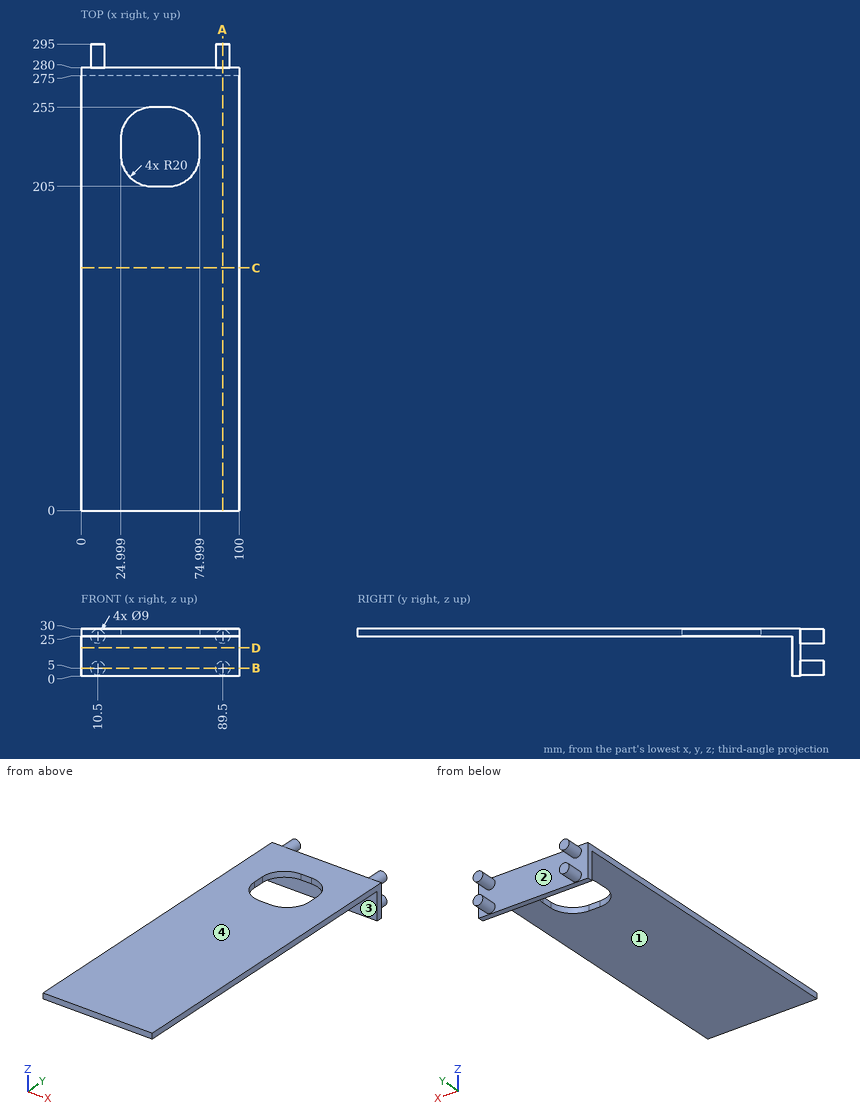
Study the drawing (mm; zero at the part's minimum x, y, z) and answer. A direction names the side the tool comes from. Round coordinates to 2 decimals unless told otherwise and drop trailing zeros. Write each loop counter-clockwise with the first axis right and the second up, starting at its lowest first coordinate (ties: lowest second). Pieces come first, ordered by that corner, then holes. Notation, with made-up numbers: (8, 16.5) -> (37, 16.5) arc R26 cw to (37, 55.5) -> close; hole circle Ø6 at (24.5, -28.5). An arc over 180 degrees is marked (long way). Write item = value, one per line.
1) Straight lines are drawn through the part: line 1 along Y through (x, z) = (51, 26.5); line 2 along X through (y, z) = (227.5, 28.75); line 3 along Z through (x, y) = (91.5, 106). For each, find the intervals that lie inside material, in ascending order. Write a range as [from, to].
Check values:
line_1 = [0, 205], [255, 280]
line_2 = [0, 25], [75, 100]
line_3 = [25, 30]
2) Section C-C on y = 153.5 is taken. Write down the section's boundary in (x, z).
Check values:
outline = (0, 25) -> (100, 25) -> (100, 30) -> (0, 30) -> close
3) Section B-B on z = 5 is taken. Write down the section's boundary in (x, y), plus the area to 3 significant figures.
Check values:
outline = (0, 275) -> (100, 275) -> (100, 280) -> (94, 280) -> (94, 295) -> (85, 295) -> (85, 280) -> (15, 280) -> (15, 295) -> (6, 295) -> (6, 280) -> (0, 280) -> close
area = 770 mm²
4) Given pin 1 (2 mm diameter, centred on x = 53.5, y = 34, fed in from -Z); pin 2 (8 mm diameter, centred on x = 33.5, z = 15, fed in from +Y); pin 3 (10 mm diameter, centred on x = 37.5, z = 5.5, fed in from -Y), each flat-ended and moving along its own axis, determine where each tip first touches the part or whether it passes through.
Check values:
pin_1 = 25
pin_2 = 280
pin_3 = 275
5) For a pull along X with two mould halves and no side action, classify the marked faces 1 and 2 as released by +X, released by -X, zero draft, split by the parting line, or undercut.
Check values:
face_1 = zero draft
face_2 = undercut
6) Section D-D on z = 17.75 is taken. Write down the section's boundary in (x, y), plus the area to 3 significant figures.
Check values:
outline = (0, 275) -> (100, 275) -> (100, 280) -> (0, 280) -> close
area = 500 mm²
7) Section A-A on x = 89.5 is taken. Write down the section's boundary in (y, z).
Check values:
outline = (0, 25) -> (275, 25) -> (275, 0) -> (280, 0) -> (280, 0.5) -> (295, 0.5) -> (295, 9.5) -> (280, 9.5) -> (280, 20.5) -> (295, 20.5) -> (295, 29.5) -> (280, 29.5) -> (280, 30) -> (0, 30) -> close
8) Which of the six approach directions +Z, -Z, +X, -X, +Y, -Y give full straight-line access (tool end or side, diameter ignored) to the marked faces 3 and 4?
Check values:
face_3 = -Z, +X, -X, -Y
face_4 = +Z, +X, -X, +Y, -Y
